Design review of the part built by this model. Coordinates are the model's own, in mm. A direction names the side the tool comes from. Coordinates: 2 decimals unless noted, no trailing zeros. Write each loop counter-clockwise with the first axis right and the second up, starting at its lowest first coordinate (ties: lowest second). Pieces come first, ordered by that corner, then holes. Notation, with made-up numbers: (13, -4.75) - (29, -4.75) arc R16 cw to (29, 17.25) - close; hole circle Ø3 at (38.5, 25.5). An arc over 180 degrees is marked (long way). Use a Markdown table: item, result.
Solid Edge part; units mm, degrees
sketch "Sketch1" plane through (0, 0, 0) normal (1, 0, 0) x (0, 1, 0)
  line L0 (0, 0) -> (19, 0)
  line L1 (19, 0) -> (19, -3)
  arc A0 (19, -3) -> (17, -5) centre (17, -3) cw
  line L2 (17, -5) -> (7.75, -5)
  line L3 (7.75, -28) -> (7.75, -5)
  line L4 (7.75, -28) -> (0, -28)
  line L5 (0, 0) -> (0, -28)
revolve "RevolvedProtrusion1" add sketch "Sketch1" angle 360 about axis through (0, 0, 0) along (0, 0, 1)
sketch "Sketch2" plane through (0, 0, -28) normal (0, 0, -1) x (0, 1, 0)
  circle A0 centre (0, 0) radius 6.15
extrude "Cutout1" cut sketch "Sketch2" against normal blind 25
fillet "Lekerekítés_1" radius 2 1 edges at (-7.75, 0, -28)
properties material "Polipropilén, általános rendeltetésű"
(1) Draft analysis for pull direction Y (two halves, no side actions). For faces 1 (the flat face through (0, 0, -3)), 2 (the flat face through (0, 0, 0)), 3 (the cylindrical face through (-6.004, -1.333, -15.675)), 4 (the cylindrical face through (-7.684, -1.009, -15.373)), state which applies: +Y half, -Y half, draft (parallel to the pull), parting line (faces both ways), or undercut.
Determined:
| item | result |
|---|---|
| face 1 | undercut |
| face 2 | draft |
| face 3 | undercut |
| face 4 | parting line |
(2) For pin 1 (5 mm diameter, centred on x = 2, z = -22.5, fed in from +Y); pin 2 (4 mm diameter, centred on x = -4, z = -17, fed in from +Y); pin 3 (12 mm diameter, centred on x = -1.5, z = -23.5, fed in from -Y), all flat-tipped, find the tip position at first contact; note any pin that passes through.
Determined:
| item | result |
|---|---|
| pin 1 | y = 7.75 |
| pin 2 | y = 7.49 |
| pin 3 | y = -7.75 |
(3) Take a section at C-C on z = -8. Write out the cut boundary in (x, y).
Determined:
| item | result |
|---|---|
| outline | circle Ø15.5 at (0, 0); hole circle Ø12.3 at (0, 0) |
(4) Machinability: for faces 5 (the cylindrical face through (-16.856, 8.767, -1.521)), 6 (the flat face through (4, 7, -5)), which of the approach directions +Z, -Z, +X, -X, +Y, -Y give a long, thin tool a straight path to every point of the face, cutting with its end or side? Answer none if there is none.
Determined:
| item | result |
|---|---|
| face 5 | +Z, -Z |
| face 6 | -Z |
(5) Take a section at A-A on y = 0. Write out the cut boundary in (x, z), and give its area (3 significant figures).
Determined:
| item | result |
|---|---|
| outline | (-19, -3) arc R2 ccw to (-17, -5) - (-7.75, -5) - (-7.75, -26.04) arc R2 ccw to (-6.15, -28) - (-6.15, -3) - (6.15, -3) - (6.15, -28) arc R2 ccw to (7.75, -26.04) - (7.75, -5) - (17, -5) arc R2 ccw to (19, -3) - (19, 0) - (-19, 0) - close |
| area | 236 mm2 |
(6) For L1, parallel to X at y = 0, z = -20; L2, parallel to Z at x = -0.5, y = 9.5; L3, parallel to X at y = -2, z = -10, list the stretches that pass through material, from the lowest coordinate up. Write a range as from..to.
Determined:
| item | result |
|---|---|
| L1 | -7.75..-6.15, 6.15..7.75 |
| L2 | -5..0 |
| L3 | -7.49..-5.82, 5.82..7.49 |
